Read the model definition and answer for the solid it produces. Units are mm, in the model's axes. A direction names the side the tool comes from. Coordinates: 2 decimals unless noted, no trailing zeros. Write each loop counter-clockwise with the first axis right and the second up, starting at its lowest first coordinate (ties: lowest second). Pieces come first, ordered by that corner, then holes.
(1) Section B-B on z = 0.9 is taken. Write down the section's boundary in (x, y), then the cut area to 3 significant figures.
(2) Section A-A on y = 2.75 is taken. Write down the section's boundary in (x, z), then the cut area to 3 significant figures.
(3) Which of the six approach directions +Z, -Z, +X, -X, +Y, -Y give full straight-line access (tool end or side, diameter ignored) to faces 4 (the flat face through (54, 0, 2)), 5 (the flat face through (1, 9, 0)), 6 (the flat face through (55.7, 5, -1))?
(4) Find the intervals of material crossed by probe 1 along X at (y, z) = (11.75, 0.4), in increasing order.
(5) The mould has two halves that part along Y. Classify faces 1 (the flat face through (27, 18, 0)), 2 (the flat face through (27, -4, 0)), 3 (the flat face through (3, 9, 1)): +Y half, -Y half, draft (parallel to the pull), parting line (faces both ways), or undercut.
(6) Given pin 1 (2 mm diameter, centred on y = 6, z = 1.5, fed in from -X); pin 2 (0.9 mm diameter, centred on x = 53.5, z = 1.5, fed in from +Y); pin 3 (0.9 mm diameter, centred on x = 54.5, y = 11.5, fed in from +Z), each flat-ended and moving along its own axis, determine where each tip first touches the part or whether it passes through.
from build123d import *

# Parameters (mm, degrees)
EXTRUDE_1_DEPTH = 18
SKETCH_2_W      = 55.7
SKETCH_2_H      = 6
EXTRUDE_2_DEPTH = 4


with BuildPart() as part:
    # 草图1 → 凸台-拉伸1 (new body)
    with BuildSketch(Plane(origin=(0, 0, 0), x_dir=(1, 0, 0), z_dir=(0, 1, 0))):
        Polygon((0, 0), (3, 0), (3, -3), (52.7, -3), (52.7, 0), (55.7, 0), (55.7, 3), (0, 3), align=None)
    extrude(amount=EXTRUDE_1_DEPTH)

    # 草图2 → 凸台-拉伸2 (add)
    with BuildSketch(Plane.XZ):
        with Locations((27.85, 0)):
            Rectangle(SKETCH_2_W, SKETCH_2_H)
    extrude(amount=EXTRUDE_2_DEPTH)


solid = part.part
Response:
1. outline: (0, -4) - (55.7, -4) - (55.7, 0) - (52.7, 0) - (52.7, 18) - (3, 18) - (3, 0) - (0, 0) - close
1. area: 1,120 mm2
2. outline: (0, -3) - (55.7, -3) - (55.7, 0) - (52.7, 0) - (52.7, 3) - (3, 3) - (3, 0) - (0, 0) - close
2. area: 316 mm2
3. face 4: +Z, +X, +Y
3. face 5: +Z, -X, +Y
3. face 6: +Z, -Z, +X, +Y, -Y
4. probe 1: x = 3 to 52.7
5. face 1: +Y half
5. face 2: -Y half
5. face 3: draft
6. pin 1: stops at x = 3
6. pin 2: stops at y = 0
6. pin 3: stops at z = 0
